```python
from build123d import *

# Parameters (mm, degrees)
F0_W     = 7.9375
F0_H     = 155.575
F1_DEPTH = 3.175
F2_R     = 1.7272
F3_DEPTH = 3.175
F4_R     = 3.96874


# Not quite as in the source:
# - a fillet or chamfer is up to 0.001 mm smaller than in the source, because OpenCascade refuses the exact size


with BuildPart() as f1:
    # F0 (on Top) → F1 (new body)
    with BuildSketch(Plane.XY):
        Rectangle(F0_W, F0_H)
    extrude(amount=F1_DEPTH)

    # F2 (on face) → F3 (cut, through all)
    with BuildSketch(Plane.XY.offset(3.175)):
        with Locations((0, 73.81875)):
            Circle(F2_R)
        with Locations((0, -73.81875)):
            Circle(F2_R)
    extrude(amount=-F3_DEPTH, mode=Mode.SUBTRACT)

    # F4 (radius 3.96875 in the source; OpenCascade refuses exactly that, so slightly less here)
    f4_edges = [f1.edges().sort_by_distance(p)[0] for p in [
        (-3.96875, -77.7875, 1.5875),
        (3.96875, -77.7875, 1.5875),
        (3.96875, 77.7875, 1.5875),
        (-3.96875, 77.7875, 1.5875),
    ]]
    fillet(f4_edges, radius=F4_R)


solid = f1.part
```
The model under review builds one solid part; all positions refer to its coordinate system, in mm. Give positions to 0.01 mm unless a question says otherwise; leave off trailing zeros. Answer in a Markdown table with one row per item.
Item 1: For line 1 along Y through (x, z) = (1.5, 1.75); line 2 along Y through (x, z) = (0.5, 1.7); line 3 along Y through (x, z) = (-3, 1.95), list the stretches that pass through material, from the lowest coordinate up.
Check sheet entries:
| item | result |
|---|---|
| line 1 | -77.49 to -74.68, -72.96 to 72.96, 74.68 to 77.49 |
| line 2 | -77.76 to -75.47, -72.17 to 72.17, 75.47 to 77.76 |
| line 3 | -76.42 to 76.42 |
Item 2: Add section A-A on z = 2.5. State how many separate pieces and enclosed holes the cut face has, plus the area to 3 significant figures.
Check sheet entries:
| item | result |
|---|---|
| separate pieces | 1 |
| enclosed holes | 2 |
| area | 1,200 mm2 |
Item 3: For P1, Ø3, axis at x = 1, y = 46, coming from the -Z side; P2, Ø1.5, axis at x = 3, z = 3, coming from the +Y side; P3, Ø1, axis at x = 2, z = 0.5, coming from the +Y side; P4, Ø3, axis at x = 0, y = -73.82, coming from the +Z side, all flat-tipped, find the tip position at first contact; note any pin that passes through.
Check sheet entries:
| item | result |
|---|---|
| P1 | z = 0 |
| P2 | y = 77.09 |
| P3 | y = 77.49 |
| P4 | through |
Item 4: Draft analysis for pull direction X (two halves, no side actions). For faces 1 (the face through (-2.84, -76.59, 1.61)), 2 (the face through (0.8, -75.35, 1.61)), 3 (the face through (0, 1, 3.175)), state which applies: +X half, -X half, draft (parallel to the pull), parting line (faces both ways), or undercut.
Check sheet entries:
| item | result |
|---|---|
| face 1 | -X half |
| face 2 | undercut |
| face 3 | draft |
